The listing builds one solid part. Answer for the finished solid, in the listing's coordinates (mm). Give positions to 0.01 mm unless a question says otherwise; leave off trailing zeros. Order: outer loops, then holes, each group sorted by start corner. A loop starts at its lowest first (then second) coordinate and runs counter-clockwise, first axis right, second up.
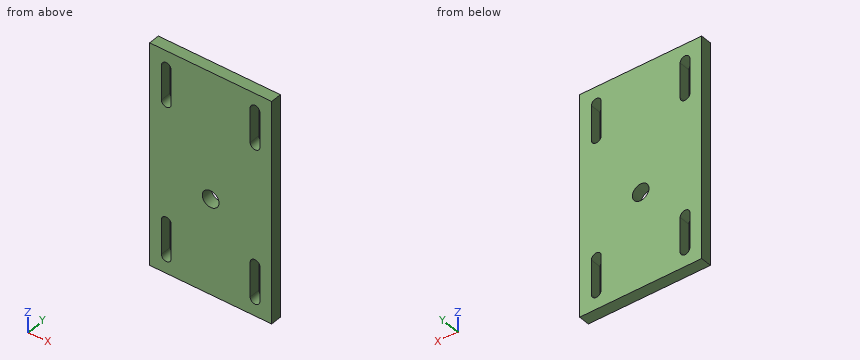
```python
from build123d import *

# Parameters (mm, degrees)
F0_W     = 139.7
F0_H     = 254
F1_DEPTH = 12.7
F2_R     = 9.525
F3_DEPTH = 25.4


with BuildPart() as f1:
    # F0 (on Front) → F1 (new body)
    with BuildSketch(Plane.XZ):
        Rectangle(F0_W, F0_H)
        with BuildLine():
            Line((-56.356148, -107.916253), (-56.35625, -68.262514))
            ThreePointArc((-56.35625, -68.262514), (-50.8, -62.70625), (-45.24375, -68.262514))
            Line((-45.24375, -68.262514), (-45.24375, -107.95))
            ThreePointArc((-45.24375, -107.95), (-50.783112, -113.506224), (-56.356147, -107.983775))
            Line((-56.356147, -107.983775), (-56.356148, -107.916253))
        make_face(mode=Mode.SUBTRACT)
        with BuildLine():
            ThreePointArc((45.24375, -68.262514), (50.8, -62.70625), (56.35625, -68.262514))
            Line((56.35625, -68.262514), (56.356148, -107.916253))
            Line((56.356148, -107.916253), (56.356147, -107.983775))
            ThreePointArc((56.356147, -107.983775), (50.783112, -113.506224), (45.24375, -107.95))
            Line((45.24375, -107.95), (45.24375, -68.262514))
        make_face(mode=Mode.SUBTRACT)
        with BuildLine():
            ThreePointArc((-56.356147, 107.983775), (-50.783112, 113.506224), (-45.24375, 107.95))
            Line((-45.24375, 107.95), (-45.24375, 68.262514))
            ThreePointArc((-45.24375, 68.262514), (-50.8, 62.70625), (-56.35625, 68.262514))
            Line((-56.35625, 68.262514), (-56.356148, 107.916253))
            ThreePointArc((-56.356148, 107.916253), (-56.35625, 107.950014), (-56.356147, 107.983775))
        make_face(mode=Mode.SUBTRACT)
        with BuildLine():
            Line((45.24375, 68.262514), (45.24375, 107.95))
            ThreePointArc((45.24375, 107.95), (50.783112, 113.506224), (56.356147, 107.983775))
            ThreePointArc((56.356147, 107.983775), (56.35625, 107.950014), (56.356148, 107.916253))
            Line((56.356148, 107.916253), (56.35625, 68.262514))
            ThreePointArc((56.35625, 68.262514), (50.8, 62.70625), (45.24375, 68.262514))
        make_face(mode=Mode.SUBTRACT)
    extrude(amount=F1_DEPTH)

    # F2 (on face) → F3 (cut)
    with BuildSketch(Plane.XZ.offset(12.7)):
        with Locations((0, -17.903471)):
            Circle(F2_R)
    extrude(amount=-F3_DEPTH, mode=Mode.SUBTRACT)


solid = f1.part
```
1) Find section A-A (x = -50.8). Write down the section's boundary in (y, z), then the cut area to 3 significant figures.
Geometry says:
outline: (-12.7, -127) - (0, -127) - (0, -113.51) - (-12.7, -113.51) - close; (-12.7, -62.71) - (0, -62.71) - (0, 62.71) - (-12.7, 62.71) - close; (-12.7, 113.51) - (0, 113.51) - (0, 127) - (-12.7, 127) - close
area: 1,940 mm2
2) Straight lines are drawn through the part: probe 1 along X at (y, z) = (-7.5, -79); probe 2 along Z at (x, y) = (0, -4); probe 3 along X at (y, z) = (-4, 109.5). For each, find the intervals that lie inside material, in ascending order.
Geometry says:
probe 1: x = -69.85 to -56.36, -45.24 to 45.24, 56.36 to 69.85
probe 2: z = -127 to -27.43, -8.38 to 127
probe 3: x = -69.85 to -56.14, -45.46 to 45.46, 56.14 to 69.85
3) Find section B-B (z = -21). Write down the section's boundary in (x, y), then the cut area to 3 significant figures.
Geometry says:
outline: (-69.85, -12.7) - (-9.01, -12.7) - (-9.01, 0) - (-69.85, 0) - close; (9.01, -12.7) - (69.85, -12.7) - (69.85, 0) - (9.01, 0) - close
area: 1,550 mm2
4) Find section C-C (x = 0). Write down the section's boundary in (y, z), then the cut area to 3 significant figures.
Geometry says:
outline: (-12.7, -127) - (0, -127) - (0, -27.43) - (-12.7, -27.43) - close; (-12.7, -8.38) - (0, -8.38) - (0, 127) - (-12.7, 127) - close
area: 2,980 mm2
5) Find section D-D (z = -88). Write down the section's boundary in (x, y), then the cut area to 3 significant figures.
Geometry says:
outline: (-69.85, -12.7) - (-56.36, -12.7) - (-56.36, 0) - (-69.85, 0) - close; (-45.24, -12.7) - (45.24, -12.7) - (45.24, 0) - (-45.24, 0) - close; (56.36, -12.7) - (69.85, -12.7) - (69.85, 0) - (56.36, 0) - close
area: 1,490 mm2
